from build123d import *

# Parameters (mm, degrees)
F1_DEPTH      = 29
F2_R          = 3
F3_W          = 30
F3_H          = 11
F4_DEPTH      = 63.5010001
F4_DEPTH_BACK = 63.5010001
F6_DEPTH      = 27.001


with BuildPart() as f1:
    # F0 (on Front) → F1 (new body, symmetric)
    with BuildSketch(Plane.XZ):
        with BuildLine():
            Line((-52.5, 0), (52.5, 0))
            Line((52.5, 0), (52.5, 9))
            Line((52.5, 9), (63.5, 9))
            ThreePointArc((63.5, 9), (55.0060966544, 29.5060966544), (34.5, 38))
            Line((34.5, 38), (-34.5, 38))
            ThreePointArc((-34.5, 38), (-55.0060966544, 29.5060966544), (-63.5, 9))
            Line((-63.5, 9), (-52.5, 9))
            Line((-52.5, 9), (-52.5, 0))
        make_face()
    extrude(amount=F1_DEPTH, both=True)

    # F2
    f2_edges = [f1.edges().sort_by_distance(p)[0] for p in [
        (0, -29, 38),
        (0, 29, 38),
    ]]
    fillet(f2_edges, radius=F2_R)

    # F3 (on Right) → F4 (cut, two sides)
    with BuildSketch(Plane.YZ) as f4_sk:
        with Locations((0, 32.5)):
            Rectangle(F3_W, F3_H)
    extrude(amount=-F4_DEPTH, mode=Mode.SUBTRACT)
    extrude(f4_sk.sketch, amount=F4_DEPTH_BACK, mode=Mode.SUBTRACT)

    # F5 (on face) → F6 (cut, through all)
    with BuildSketch(Plane.XY.offset(27)):
        with BuildLine():
            Line((-19.5, 6.5), (-38.5, 6.5))
            ThreePointArc((-38.5, 6.5), (-45, 0), (-38.5, -6.5))
            Line((-38.5, -6.5), (-19.5, -6.5))
            ThreePointArc((-19.5, -6.5), (-13, 0), (-19.5, 6.5))
        make_face()
        with BuildLine():
            Line((38.5, 6.5), (19.5, 6.5))
            ThreePointArc((19.5, 6.5), (13, 0), (19.5, -6.5))
            Line((19.5, -6.5), (38.5, -6.5))
            ThreePointArc((38.5, -6.5), (45, 0), (38.5, 6.5))
        make_face()
    extrude(amount=-F6_DEPTH, mode=Mode.SUBTRACT)


solid = f1.part
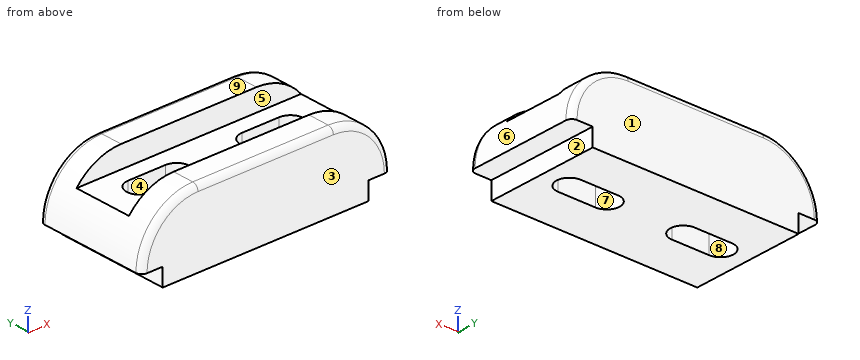
Can you work these out from the model? Positions are in its coordinate system, mm. Face numbers are marked on the shaded views. A direction names the side the tool comes from. Round coordinates to 2 decimals unless told otherwise and drop trailing zeros. Loops run counter-clockwise (first coordinate to the right, second up) from the corner with the lowest first, then second, coordinate; pieces in that order, holes last. Notation, with made-up numbers: (2, -7.5) - (13, -7.5) arc R11 cw to (13, 13.5) - close; hole circle Ø1 at (13.25, 25). An arc over 180 degrees is marked (long way). Use CSV: the item, a comma, the result in double quotes. Start each with the question number.
1) For pin 1 Ø4 at (y, z) = (1, 30.5) entering from -X; pin 2 Ø6 at (x, y) = (-47, -10.5) entering from +Z; pin 3 Ø5.5 at (x, y) = (-55.5, -0.5) entering from -Z, each with a flat end and sliding along its axis, tell me the tip position at first contact or that it passes through.
2) If we section it at D-D on x = 30.5: Write out the boundary of the cut face in (y, z).
3) If we section it at A-A on y = 0: Write out the boundary of the cut face in (x, z).
4) We'd pull the mould along X, two halves only. Please class the marked faces 6, 7, 8 and 9: released by +X, released by -X, zero draft, split by the parting line, or undercut.
5) Please list where these lines run through material, in increasing order: probe 1 along Y at (x, z) = (9.5, 33.5); probe 2 along X at (y, z) = (4, 4.5); probe 3 along Y at (x, z) = (-32, 24.5). Write a range as [from, to].
6) If we section it at C-C on y = -13.5: Write out the boundary of the cut face in (x, z), plus the area to 3 significant figures.
7) For the marked faces 1, 2, 3, 4 and 5, which set-ups out of +Z, -Z, +X, -X, +Y, -Y let a thin tool reach every point of the face, with its end or its side?
8) If we section it at B-B on x = -0.5: Write out the boundary of the cut face in (y, z).
Geometry results:
1,pin 1,"passes through"
1,pin 2,"stops at z = 27"
1,pin 3,"stops at z = 9"
2,outline,"(-29, 0) - (-6.5, 0) - (-6.5, 27) - (-15, 27) - (-15, 38) - (-26, 38) arc R3 ccw to (-29, 35) - close; (6.5, 0) - (29, 0) - (29, 35) arc R3 ccw to (26, 38) - (15, 38) - (15, 27) - (6.5, 27) - close"
3,outline,"(-63.5, 9) - (-52.5, 9) - (-52.5, 0) - (-45, 0) - (-45, 27) - (-57.24, 27) arc R29 ccw to start; (-13, 0) - (13, 0) - (13, 27) - (-13, 27) - close; (45, 0) - (52.5, 0) - (52.5, 9) - (63.5, 9) arc R29 ccw to (57.24, 27) - (45, 27) - close"
4,face 6,"released by +X"
4,face 7,"undercut"
4,face 8,"undercut"
4,face 9,"zero draft"
5,probe 1,"y = [-29, -15], [15, 29]"
5,probe 2,"x = [-52.5, -43.62], [-14.38, 14.38], [43.62, 52.5]"
5,probe 3,"y = [-29, -6.5], [6.5, 29]"
6,outline,"(-63.5, 9) - (-52.5, 9) - (-52.5, 0) - (52.5, 0) - (52.5, 9) - (63.5, 9) arc R29 ccw to (57.24, 27) - (-57.24, 27) arc R29 ccw to start"
6,area,"3,160 mm2"
7,face 1,"+Z, -Z, +X, -X, +Y"
7,face 2,"-Z, +X, +Y, -Y"
7,face 3,"+Z, -Z, +X, -X, -Y"
7,face 4,"+Z, -Z"
7,face 5,"+Z, +X, -X"
8,outline,"(-29, 0) - (29, 0) - (29, 35) arc R3 ccw to (26, 38) - (15, 38) - (15, 27) - (-15, 27) - (-15, 38) - (-26, 38) arc R3 ccw to (-29, 35) - close"
